The model under review builds one solid part; all positions refer to its coordinate system, in mm. Round coordinates to 2 decimals unless told otherwise and drop trailing zeros. Loops run counter-clockwise (first coordinate to the right, second up) from the corner with the lowest first, then second, coordinate; pieces in that order, holes last. Notation, with made-up numbers: (71, 12.5) -> (123, 12.5) arc R10 ccw to (123, 29.5) -> close; hole circle Ø4 at (38.5, 18). An arc over 180 degrees is marked (long way). Use a Markdown table: item, result. Add a question column.
1) Consider section D-D on x = 1.25. Give the boundary of the cut face in (y, z), plus the area to 3 significant figures.
2) Consider section A-A on y = -50. State how many separate pieces and enclosed holes the cut face has, plus the area to 3 significant figures.
3) Consider section C-C on y = -30. Give the boundary of the cut face in (x, z), plus the area to 3 significant figures.
4) Wall thickness on probe 1 along Y at (x, z) = (1.1, -11); probe 2 along Z at (x, y) = (0.9, -29); probe 3 along Y at (x, z) = (0.7, -36): over which ranges is each line inside the solid? List them lowest first.
5) Consider section B-B on z = -30. Give the boundary of the cut face in (x, y), plus the area to 3 significant figures.
6) Mouldability with a two-part tool opening along Z and no side actions: class faces 1 (the conical face through (1.87, -51.88, -11.41)), 2 (the conical face through (0.14, -59.15, -0.83)), 3 (the flat face through (4, -36, -23)), 4 (the flat face through (2, -20, -40)) as released by +Z, released by -Z, zero draft, split by the parting line, or undercut.
7) Insertion check: pin 1 (3.5 mm diameter, centred on y = -50, z = -50, fed in from +X). The pin has a flat end and moves straight along its axis. Give the tip position at first contact, or say it passes through.
Autodesk Fusion 360 part; units mm, degrees
sketch "Sketch1" plane through (0, 0, 0) normal (1, 0, 0) x (0, 0, -1)
  line L0 (0, 0) -> (0, -60)
  line L1 (0, -60) -> (60, -60)
  line L2 (60, -60) -> (60, -40)
  line L3 (20, 0) -> (0, 0)
  line L4 (60, -40) -> (40, -20)
  line L5 (60, -50) -> (0, -50) construction
  line L6 (10.2088, 0) -> (10.2088, -60) construction
  line L7 (0, -9.7462) -> (40, -10) construction
  line L8 (0, -30) -> (50, -30) construction
  line L9 (49.9986, -60) -> (50, -30) construction
  line L10 (30, -60) -> (30, 0) construction
  circle A0 centre (10.2088, -9.811) radius 2.1
  circle A1 centre (10.2088, -30) radius 2.1
  circle A2 centre (10.2088, -50) radius 2.1
  circle A3 centre (30, -50) radius 2.1
  circle A4 centre (49.9991, -50) radius 2.1
  line L11 (60, -40) -> (20, 0)
  dimension "d1" = 60
  dimension "d2" = 60
  dimension "d3" = 20
  dimension "d15" = 4.2
  dimension "d16" = 4.2
  dimension "d17" = 4.2
  dimension "d18" = 4.2
  dimension "d19" = 4.2
extrude "Extrude1" add sketch "Sketch1" along normal blind 4
chamfer "Chamfer1" distance 2 angle 45 5 edges at (0, -9.0516, -8.2509) (0, -29.2406, -8.2509) (0, -49.2406, -8.2509) (0, -49.2406, -28.0421) (0, -49.2406, -48.0412)
fillet "Fillet1" radius 2 4 edges at (2, -60, -60) (2, -60, 0) (2, -40, -60) (2, 0, 0)
chamfer "Chamfer2" distance 0.5 angle 45 17 edges at (0, -60, -30) (0, -59.4142, -59.4142) (0, -49.4142, -60) (0, -40.0631, -59.8478) (0, -19.7071, -39.7071) (0, 0, -11) (0, -0.5858, -0.5858) (0, -30, 0) (4, -19.7071, -39.7071) (4, -40.0631, -59.8478) (4, -49.4142, -60) (4, -59.4142, -59.4142) (4, -60, -30) (4, -59.4142, -0.5858) (4, -30, 0) (4, -0.5858, -0.5858) (4, 0, -11)
chamfer "Chamfer3" distance 0.2 angle 45 5 edges at (4, -9.0516, -8.2509) (4, -29.2406, -8.2509) (4, -49.2406, -8.2509) (4, -49.2406, -28.0421) (4, -49.2406, -48.0412)
Result set:
| question | item | result |
|---|---|---|
| 1 | outline | (-60, -58) arc R2 ccw to (-58, -60) -> (-40.83, -60) arc R2 ccw to (-39.41, -59.41) -> (0, -20) -> (0, -2) arc R2 ccw to (-2, 0) -> (-58, 0) arc R2 ccw to (-60, -2) -> close; hole circle Ø5.7 at (-50, -50); hole circle Ø5.7 at (-50, -30); hole circle Ø5.7 at (-50, -10.21); hole circle Ø5.7 at (-30, -10.21); hole circle Ø5.7 at (-9.81, -10.21) |
| 1 | area | 2,670 mm2 |
| 2 | separate pieces | 4 |
| 2 | enclosed holes | 0 |
| 2 | area | 177 mm2 |
| 3 | outline | (0, -49.29) -> (0.5, -50) -> (3.5, -50) -> (4, -49.29) -> (4, -12.51) -> (3.8, -12.31) -> (2, -12.31) -> (0, -14.31) -> close; (0, -6.11) -> (2, -8.11) -> (3.8, -8.11) -> (4, -7.91) -> (4, -0.5) -> (3.5, 0) -> (0.5, 0) -> (0, -0.5) -> close |
| 3 | area | 179 mm2 |
| 4 | probe 1 | -60 to -52.89, -47.11 to -32.89, -27.11 to -12.7, -6.92 to 0 |
| 4 | probe 2 | -49 to -13.25, -7.17 to 0 |
| 4 | probe 3 | -60 to -16 |
| 5 | outline | (0, -59.5) -> (0.5, -60) -> (3.5, -60) -> (4, -59.5) -> (4, -52.3) -> (3.8, -52.1) -> (2, -52.1) -> (0, -54.1) -> close; (0, -45.9) -> (2, -47.9) -> (3.8, -47.9) -> (4, -47.7) -> (4, -10.71) -> (3.5, -10) -> (0.5, -10) -> (0, -10.71) -> close |
| 5 | area | 179 mm2 |
| 6 | face 1 | undercut |
| 6 | face 2 | released by +Z |
| 6 | face 3 | zero draft |
| 6 | face 4 | released by -Z |
| 7 | pin 1 | through |
